Solid Edge part; units mm, degrees
sketch "Sketch1" plane through (0, 0, 0) normal (1, 0, 0) x (0, 1, 0)
  line L0 (-70.6829, -67.8929) -> (-40.6829, -67.8929)
  line L1 (-40.6829, -67.8929) -> (-40.6829, 12.1071)
  line L2 (-40.6829, 12.1071) -> (-70.6829, 12.1071)
  line L3 (-70.6829, 12.1071) -> (-70.6829, -67.8929)
  line L4 (-70.6829, 12.1071) -> (-40.6829, 12.1071)
  line L5 (-54.1753, 28.1984) -> (-40.6829, 12.1071)
  line L6 (-57.1901, 28.1988) -> (-54.1753, 28.1984)
  line L7 (-70.6829, 12.1071) -> (-57.1901, 28.1988)
  dimension "D1" = 70.6829
  dimension "D2" = 54.1753
  dimension "D3" = 70.6829
  dimension "D4" = 40.6829
  dimension "D5" = 40.6829
  dimension "D6" = 0
extrude "Protrusion1" add sketch "Sketch1" against normal blind 3
sketch "Sketch2" plane through (0, -21.8205, 20.1807) normal (1, 0, 0) x (0, 1, 0)
  circle A0 centre (-33.8621, -1.9821) radius 5
  dimension "D1" = 33.8621
  dimension "D2" = 33.8621
extrude "ExtrudedProtrusion_2" add sketch "Sketch2" along normal blind 11
mirror "Mirror1" about plane through (5, -21.8205, 20.1506) normal (1, 0, 0) of "Protrusion1"
sketch "Sketch3" plane through (11.5, -70.6829, -27.8929) normal (0, -1, 0) x (0, 0, -1)
  arc A0 (40, -1.5) -> (40, -11.5) centre (88.482, -6.5) ccw
  line L0 (38.9458, -1.5) -> (40, -1.5)
  arc A1 (38.9458, -1.5) -> (38.9458, -11.5) centre (88.6952, -6.5) ccw
  line L1 (40, -11.5) -> (38.9458, -11.5)
extrude "ExtrudedProtrusion_4" add sketch "Sketch3" against normal blind 30
For this review, take the finished solid that the model builds, in its own axes (mm). A direction names the side the tool comes from. Coordinates: 2 decimals unless noted, no trailing zeros. Order: outer loops, then holes, each group sorted by start corner. A loop starts at its lowest first (then second) coordinate and runs counter-clockwise, first axis right, second up. Notation, with made-up numbers: (54, 12.25) - (113, 12.25) arc R27 cw to (113, 43.25) - close; hole circle Ø2 at (-30, 55). An arc over 180 degrees is marked (long way). Use one line per item in the form item = value.
Q1. Consider section B-B (x = 7). Give the boundary of the cut face in (y, z), then the cut area to 3 significant figures.
Checked values:
outline = (-70.68, -67.68) - (-40.68, -67.68) - (-40.68, -66.63) - (-70.68, -66.63) - close; circle Ø10 at (-55.68, 18.2)
area = 110 mm2
Q2. Consider section C-C (y = -58.5). Give the boundary of the cut face in (x, z).
Checked values:
outline = (-3, -67.89) - (0, -67.89) arc R48.74 cw to (10, -67.89) - (13, -67.89) - (13, 26.64) - (10, 26.64) - (10, 22.33) - (0, 22.33) - (0, 26.64) - (-3, 26.64) - close; hole (0, -66.84) arc R50 cw to (10, -66.84) - (10, 14.07) - (0, 14.07) - close
Q3. For P1, Ø1.5, axis at x = 11, y = -59.5, coming from the +Z side, flat-tipped, find the tip position at first contact; note if it passes through.
Checked values:
P1 = 26.34
Q4. Consider section A-A (z = -29.5). Give the boundary of the cut face in (x, y), then the cut area to 3 significant figures.
Checked values:
outline = (-3, -70.68) - (0, -70.68) - (0, -40.68) - (-3, -40.68) - close; (10, -70.68) - (13, -70.68) - (13, -40.68) - (10, -40.68) - close
area = 180 mm2
Q5. Draft analysis for pull direction X (two halves, no side actions). For faces 1 (the flat face through (13, -56, -19)), 2 (the flat face through (0, -56, -20)), 3 (the cylindrical face through (5.07, -55.893, -67.636)), 4 (the flat face through (-1.479, -47.524, 20.265)), state which applies: +X half, -X half, draft (parallel to the pull), parting line (faces both ways), or undercut.
Checked values:
face_1 = +X half
face_2 = undercut
face_3 = undercut
face_4 = draft
Q6. For faces 5 (the cylindrical face through (4.93, -59.65, 21.24)), 6 (the flat face through (-1, -56, -67.893)), 7 (the cylindrical face through (5.07, -55.89, -66.59)), list the 3-axis set-ups (+Z, -Z, +X, -X, +Y, -Y) from which the entire face can be reached by the end or side of a thin tool; tool diameter is ignored.
Checked values:
face_5 = none
face_6 = -Z, +X, -X, +Y, -Y
face_7 = +Y, -Y
Q7. For probe 1 along X at (y, z) = (-61, 5.5); probe 2 along Z at (x, y) = (3.75, -62); probe 3 along Z at (x, y) = (1.25, -57), list the stretches that pass through material, from the lowest coordinate up. Write a range as from..to.
Checked values:
probe_1 = -3..0, 10..13
probe_2 = -67.65..-66.6
probe_3 = -67.78..-66.73, 13.38..23.02
Q8. Consider section D-D (y = -66). Give the boundary of the cut face in (x, z).
Checked values:
outline = (-3, -67.89) - (0, -67.89) arc R48.74 cw to (10, -67.89) - (13, -67.89) - (13, 17.69) - (10, 17.69) - (10, -66.84) arc R50 ccw to (0, -66.84) - (0, 17.69) - (-3, 17.69) - close
